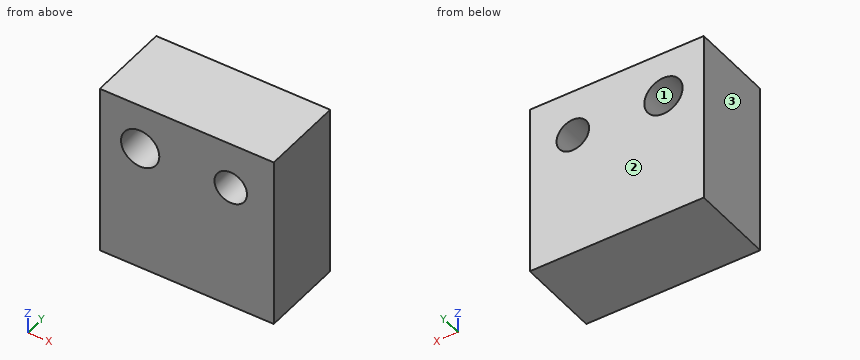
```python
from build123d import *

# Parameters (mm, degrees)
F0_W     = 52.7440756559
F0_H     = 52.2768497467
F1_DEPTH = 25.4
F2_R     = 4.8102139617
F3_DEPTH = 126.0972395539
F4_R     = 4.9351190146
F5_DEPTH = 76.2
F6_R     = 5.8080274439
F8_DEPTH = 25.4


# Not quite as in the source:
# - the program builds the solid bodies; features that only make, move or delete a surface that nothing else refers to are left out


with BuildPart() as f1:
    # F0 (on Front) → F1 (new body)
    with BuildSketch(Plane.XZ):
        with Locations((-1.0988339782, 2.8451383114)):
            Rectangle(F0_W, F0_H)
    extrude(amount=F1_DEPTH)

    # F2 (on Front) → F3 (cut)
    with BuildSketch(Plane.XZ):
        with Locations((-12.8197297454, 11.39511168)):
            Circle(F2_R)
    extrude(amount=-F3_DEPTH, mode=Mode.SUBTRACT)

    # F4 (on face) → F5 (cut)
    with BuildSketch(Plane(origin=(0, 0, 0), x_dir=(-1, 0, 0), z_dir=(0, 1, 0))):
        with Locations((-12.2308423743, 14.9360494688)):
            Circle(F4_R)
    extrude(amount=-F5_DEPTH, mode=Mode.SUBTRACT)

    # F6 (on face) → F8 (cut)
    with BuildSketch(Plane.XZ.offset(25.4)):
        with Locations((-15.2422711253, 15.1493921876)):
            Circle(F6_R)
    extrude(amount=-F8_DEPTH, mode=Mode.SUBTRACT)


solid = f1.part
```
Source: CAD feature listing. Evaluate the final solid. Frame: model axes, mm. Face numbers are marked on the shaded views. Give positions to 0.01 mm unless a question says otherwise; leave off trailing zeros. Order: outer loops, then holes, each group sorted by start corner. A loop starts at its lowest first (then second) coordinate and runs counter-clockwise, first axis right, second up. Notation, with made-up numbers: (58.5, 35.25) -> (111.5, 35.25) arc R23 ccw to (111.5, 74.25) -> close; hole circle Ø4 at (89, -15). An arc over 180 degrees is marked (long way). Use a Markdown table: item, result.
Q1. Material intervals for line 1 (X direction, y = -17.25, z = 13); line 2 (Z direction, x = -16.5, y = -13.75); line 3 (X direction, y = -19.75, z = 17), sorted ascending. Write a range as [from, to].
A:
| item | result |
|---|---|
| line 1 | [-27.47, -20.64], [-9.85, 7.69], [16.77, 25.27] |
| line 2 | [-23.29, 9.48], [20.82, 28.98] |
| line 3 | [-27.47, -20.75], [-9.74, 7.75], [16.71, 25.27] |
Q2. Section C-C (y = -12). Return the cut outline in (x, z), and give its area (3 significant figures).
A:
| item | result |
|---|---|
| outline | (-27.47, -23.29) -> (25.27, -23.29) -> (25.27, 28.98) -> (-27.47, 28.98) -> close; hole circle Ø11.62 at (-15.24, 15.15); hole circle Ø9.87 at (12.23, 14.94) |
| area | 2,570 mm^2 |
Q3. Pull-direction query (X, two-part tool) for the marked faces 1, 2 and 3; classes: +X half, -X half, draft (parallel to the pull), parting line (faces both ways), or undercut.
A:
| item | result |
|---|---|
| face 1 | undercut |
| face 2 | draft |
| face 3 | -X half |
Q4. First-contact query: P1, Ø2, axis at x = 8, z = -6, coming from the +Y side; P2, Ø8, axis at x = 12.23, z = 14.94, coming from the +Y side. Flat tips, straight axial feed; report the tip coordinate or a pass-through.
A:
| item | result |
|---|---|
| P1 | y = 0 |
| P2 | through |
Q5. Section B-B (x = 14). Return the cut outline in (y, z).
A:
| item | result |
|---|---|
| outline | (-25.4, -23.29) -> (0, -23.29) -> (0, 10.33) -> (-25.4, 10.33) -> close; (-25.4, 19.54) -> (0, 19.54) -> (0, 28.98) -> (-25.4, 28.98) -> close |
Q6. Section A-A (z = 17). Return the cut outline in (x, y).
A:
| item | result |
|---|---|
| outline | (-27.47, -25.4) -> (-20.75, -25.4) -> (-20.75, 0) -> (-27.47, 0) -> close; (-9.74, -25.4) -> (7.75, -25.4) -> (7.75, 0) -> (-9.74, 0) -> close; (16.71, -25.4) -> (25.27, -25.4) -> (25.27, 0) -> (16.71, 0) -> close |
Q7. Section D-D (x = -18.5). Return the cut outline in (y, z), and give its area (3 significant figures).
A:
| item | result |
|---|---|
| outline | (-25.4, -23.29) -> (0, -23.29) -> (0, 10.34) -> (-25.4, 10.34) -> close; (-25.4, 19.96) -> (0, 19.96) -> (0, 28.98) -> (-25.4, 28.98) -> close |
| area | 1,080 mm^2 |
